Autodesk Inventor part; units mm, degrees
ref_plane "Work Plane1" through (0, -12.5, 0) normal (0, 1, 0) x (-1, 0, 0)
ref_plane "Work Plane2" through (0, -12.5, 0) normal (0, 1, 0) x (-1, 0, 0)
ref_plane "YZ Plane" through (0, 0, 0) normal (1, 0, 0) x (0, 1, 0)
sketch "Sketch1" plane through (0, 0, 0) normal (1, 0, 0) x (0, 1, 0)
  circle A0 centre (0, 0) radius 12.5
  dimension "d0" = 25
extrude "Extrusion1" add sketch "Sketch1" along normal blind 200
ref_plane "Work Plane1" through (0, -12.5, 0) normal (0, 1, 0) x (-1, 0, 0)
sketch "Sketch2" plane through (0, -12.5, 0) normal (0, 1, 0) x (-1, 0, 0)
  line L0 (-200, 12.5) -> (-200, -12.5)
  line L1 (-200, 0) -> (-140, 0)
  circle A0 centre (-140, 0) radius 7.5
  point P0 (0, 0)
  dimension "d19" = 60
  dimension "d20" = 15
extrude "Extrusion2" cut sketch "Sketch2" along normal blind 15
sketch "Sketch3" plane through (0, 0, 0) normal (-1, 0, 0) x (0, 0, 1)
  line L0 (0, 0) -> (0, -7)
  circle A0 centre (0, -7) radius 2.5
  dimension "d9" = 7
  dimension "d10" = 5
extrude "Extrusion3" cut sketch "Sketch3" against normal blind 136
sketch "Sketch4" plane through (200, 0, 0) normal (1, 0, 0) x (0, 0, -1)
  circle A0 centre (0, 0) radius 10
  dimension "d13" = 20
extrude "Extrusion4" cut sketch "Sketch4" against normal blind 6
sketch "Sketch5" plane through (194, 0, 0) normal (1, 0, 0) x (0, 0, -1)
  circle A0 centre (0, 0) radius 4
  dimension "d16" = 8
extrude "Extrusion5" cut sketch "Sketch5" against normal blind 50
sketch "Sketch6" plane through (0, 0, 0) normal (-1, 0, 0) x (0, 0, 1)
  circle A0 centre (0, 0) radius 5
  dimension "d21" = 10
extrude "Extrusion6" cut sketch "Sketch6" against normal blind 80
fillet "Fillet1" radius 0.4 2 edges at (40, -4.8393, 1.2575) (40, -4.8393, -1.2575)
sketch "Sketch7" plane through (0, 0, 0) normal (-1, 0, 0) x (0, 0, 1)
  circle A0 centre (0, 0) radius 38.5321
extrude "Extrusion7" cut sketch "Sketch7" against normal blind 40
chamfer "Chamfer1" distance 0.4 angle 45 5 edges at (40, 5, 0) (40, -4.9016, 1.691) (40, -4.9016, -1.691) (40, -6.0616, 2.3172) (40, -9.3172, -0.9384)
ref_plane "Work Plane2" through (0, -12.5, 0) normal (0, 1, 0) x (-1, 0, 0)
sketch "Sketch8" plane through (0, -12.5, 0) normal (0, 1, 0) x (-1, 0, 0)
  circle A0 centre (-152.5, 0) radius 1.5
  line L0 (-200, 12.5) -> (-200, -12.5)
  point P0 (0, 0)
  dimension "d31" = 3
  dimension "d32" = 47.5
extrude "Extrusion8" cut sketch "Sketch8" along normal blind 10
properties part number "Dowel1"
Input: part model. Units: mm. Frame: model coordinates. A direction names the side the tool comes from. Coordinates: 2 decimals unless noted, no trailing zeros. Loops run counter-clockwise (first coordinate to the right, second up) from the corner with the lowest first, then second, coordinate; pieces in that order, holes last.
(1) First-contact query: pin 1 Ø2 at (x, z) = (132, 3.5) entering from -Y; pin 2 Ø6 at (x, y) = (116.5, -5) entering from +Z; pin 3 Ø8 at (y, z) = (-7, 0) entering from -X; pin 4 Ø1.5 at (x, z) = (138, 8.5) entering from +Y. Flat tips, straight axial feed; report the tip coordinate or a pass-through.
(2) Section A-A on z = 0. Return the cut outline in (x, y), then the cut area to 3 significant figures.
(3) Section D-D on x = 152.5. Return the cut outline in (y, z).
(4) Section B-B on y = -7. Return the cut outline in (x, z).
(5) Section C-C on x = 172. Return the cut outline in (y, z), then the cut area to 3 significant figures.
(6) Material intervals for probe 1 along Y at (x, z) = (180, 0); probe 2 along Y at (x, z) = (196.55, 0), sorted ascending.
(7) Set-up query: faces 1 (the face through (86.02, -9.44, -0.54)), 2 (the face through (194, 0.1, -4.3)), 3 (the face through (40, 6, 0)), 4 (the face through (151.114, -8.166, 0.575)). Return all of +Z, -Z, +X, -X, +Y, -Y with unobstructed straight access to the full face (end or side cutting, diameter ignored); none if empty.
(8) Pull-direction query (Y, two-part tool) for faces 5 (the face through (118.88, 11.923, -3.755)), 6 (the face through (200, -0.1, 10.2)), 7 (the face through (40.286, 5.11, 0.197)); classes: released by +Y, released by -Y, zero draft, split by the parting line, or undercut.
Data:
1. pin 1: stops at y = -12.25
1. pin 2: stops at z = 12.34
1. pin 3: stops at x = 40
1. pin 4: stops at y = 9.81
2. outline: (40, -12.5) - (132.5, -12.5) - (132.5, -9.5) - (40.4, -9.5) - (40, -9.9) - close; (40, 5.4) - (40.4, 5) - (80, 5) - (80, -4.5) - (132.5, -4.5) - (132.5, 2.5) - (144, 2.5) - (144, 4) - (194, 4) - (194, 10) - (200, 10) - (200, 12.5) - (40, 12.5) - close; (147.5, -12.5) - (151, -12.5) - (151, -4) - (147.5, -4) - close; (154, -12.5) - (200, -12.5) - (200, -10) - (194, -10) - (194, -4) - (154, -4) - close
2. area: 2,410 mm2
3. outline: (-12.41, -1.5) arc R12.5 ccw (long way) to (-12.41, 1.5) - (-3.71, 1.5) arc R4 cw (long way) to (-3.71, -1.5) - close
4. outline: (40, -10.36) - (200, -10.36) - (200, -7.14) - (194, -7.14) - (194, 7.14) - (200, 7.14) - (200, 10.36) - (40, 10.36) - (40, 2.9) - (40.4, 2.5) - (132.93, 2.5) arc R7.5 cw (long way) to (132.93, -2.5) - (40.4, -2.5) - (40, -2.9) - close; hole circle Ø3 at (152.5, 0)
5. outline: circle Ø25 at (0, 0); hole circle Ø8 at (0, 0)
5. area: 441 mm2
6. probe 1: y = -12.5 to -4, 4 to 12.5
6. probe 2: y = -12.5 to -10, 10 to 12.5
7. face 1: -X
7. face 2: +X
7. face 3: +Z, -Z, -X, +Y, -Y
7. face 4: -Y
8. face 5: split by the parting line
8. face 6: zero draft
8. face 7: undercut
